Here's how the part is built. I have some questions about the finished solid (model axes, mm). Face numbers are marked on the shaded views. A direction names the side the tool comes from. Coordinates: 2 decimals unless noted, no trailing zeros. Order: outer loops, then holes, each group sorted by start corner. A loop starts at its lowest first (then second) coordinate and runs counter-clockwise, first axis right, second up.
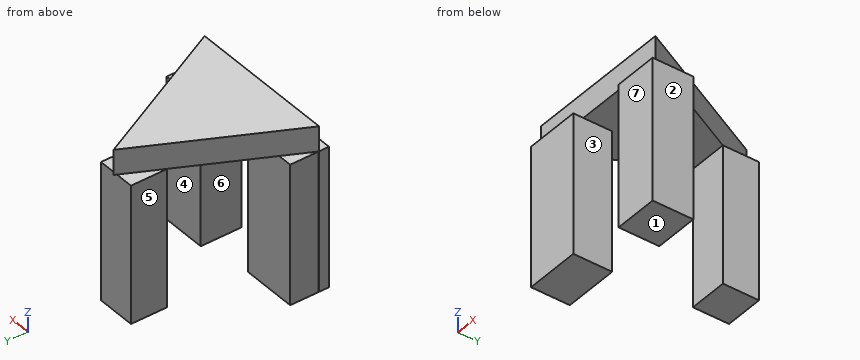
```python
from build123d import *

# Parameters (mm, degrees)
F1_DEPTH = 25.4
F4_W     = 55.9908
F4_H     = 39.370671
F5_DEPTH = 142.071173
F6_W     = 39.675076
F6_H     = 36.552988
F7_DEPTH = 139.835253
F8_W     = 45.023777
F8_H     = 41.238799
F9_DEPTH = 144.416898


with BuildPart() as f1:
    # F0 (on Top) → F1 (new body)
    with BuildSketch(Plane.XY):
        Polygon((0, 74.892037), (-75.72189, -75.514391), (75.72183, -75.306922), align=None)
    extrude(amount=F1_DEPTH)

    # F2 (on face) + F4 (on face) → F5 (join)
    with BuildSketch(Plane(origin=(0, 0, 0), x_dir=(1, 0, 0), z_dir=(0, 0, -1))):
        Polygon((-41.094646, 48.674494), (-41.094646, 75.466954), (-75.72189, 75.514391), (-62.209384, 48.674494), align=None)
    with BuildSketch(Plane(origin=(0, 0, 0), x_dir=(1, 0, 0), z_dir=(0, 0, -1))):
        with Locations((-47.557339, 65.946586)):
            Rectangle(F4_W, F4_H)
    extrude(amount=F5_DEPTH)

    # F6 (on face) → F7 (join)
    with BuildSketch(Plane(origin=(0, 0, 0), x_dir=(1, 0, 0), z_dir=(0, 0, -1))):
        with Locations((0, -54.166105)):
            Rectangle(F6_W, F6_H)
    extrude(amount=F7_DEPTH)

    # F8 (on face) → F9 (join)
    with BuildSketch(Plane(origin=(0, 0, 0), x_dir=(1, 0, 0), z_dir=(0, 0, -1))):
        with Locations((55.466999, 59.285469)):
            Rectangle(F8_W, F8_H)
    extrude(amount=F9_DEPTH)


solid = f1.part
```
Q1. If we section it at A-A on z = -84: Write out the boundary of the cut face in (x, y), then the cut area to 3 significant figures.
Q2. For the marked faces 4, 5, 6 and 7, which set-ups out of +Z, -Z, +X, -X, +Y, -Y let a thin tool reach every point of the face, with its end or its side?
Q3. We'd pull the mould along X, two halves only. Please class the marked faces 1, 2 and 3: pulls with the +X half, pulls with the -X half, needs draft (parallel to the pull), parting line crosses it, or undercut.
Q4. If we section it at B-B on y = 48.5: Write out the boundary of the cut face in (x, z).
Q5. If we section it at C-C on x = 14.5: Write out the boundary of the cut face in (y, z).
Q6. Will these pins go through, and if not, where does the flat tip stop? pin 1 (12 mm diameter, centred on x = -5, z = -58, fed in from -Y); pin 2 (10 mm diameter, centred on x = 30, z = -19.5, fed in from -Y); pin 3 (18.5 mm diameter, centred on x = 0.5, y = 45, fed in from -Z).
Q7. If we section it at D-D on z = 3.5: Write out the boundary of the cut face in (x, y), then the cut area to 3 significant figures.
Q8. I need wall thicknesses on L1, parallel to X at y = -70, z = -112; L2, parallel to Z at x = -25, y = -68.5; L3, parallel to Y at x = -54.5, z = -8. Which ranges of each line are inside material? Lowest first, please.
Reply:
1. outline: (-75.72, -75.51) - (-75.55, -75.51) - (-75.55, -85.63) - (-19.56, -85.63) - (-19.56, -46.26) - (-75.55, -46.26) - (-75.55, -75.18) - close; (-19.84, 35.89) - (19.84, 35.89) - (19.84, 72.44) - (-19.84, 72.44) - close; (32.96, -79.9) - (77.98, -79.9) - (77.98, -38.67) - (32.96, -38.67) - close
1. area: 5,510 mm2
2. face 4: -Z, +X, -X, +Y
2. face 5: +Z, -Z, -X, +Y
2. face 6: -Z, +Y, -Y
2. face 7: +Z, -Z, +X, -Y
3. face 1: needs draft
3. face 2: pulls with the +X half
3. face 3: undercut
4. outline: (-19.84, -139.84) - (19.84, -139.84) - (19.84, 0) - (13.31, 0) - (13.31, 25.4) - (-13.29, 25.4) - (-13.29, 0) - (-19.84, 0) - close
5. outline: (-75.39, 0) - (35.89, 0) - (35.89, -139.84) - (72.44, -139.84) - (72.44, 0) - (46.13, 0) - (46.13, 25.4) - (-75.39, 25.4) - close
6. pin 1: stops at y = 35.89
6. pin 2: stops at y = -79.9
6. pin 3: stops at z = -139.84
7. outline: (-75.72, -75.51) - (75.72, -75.31) - (0, 74.89) - close
7. area: 11,400 mm2
8. L1: x = -75.55 to -19.56, 32.96 to 77.98
8. L2: z = -142.07 to 25.4
8. L3: y = -85.63 to -46.26
